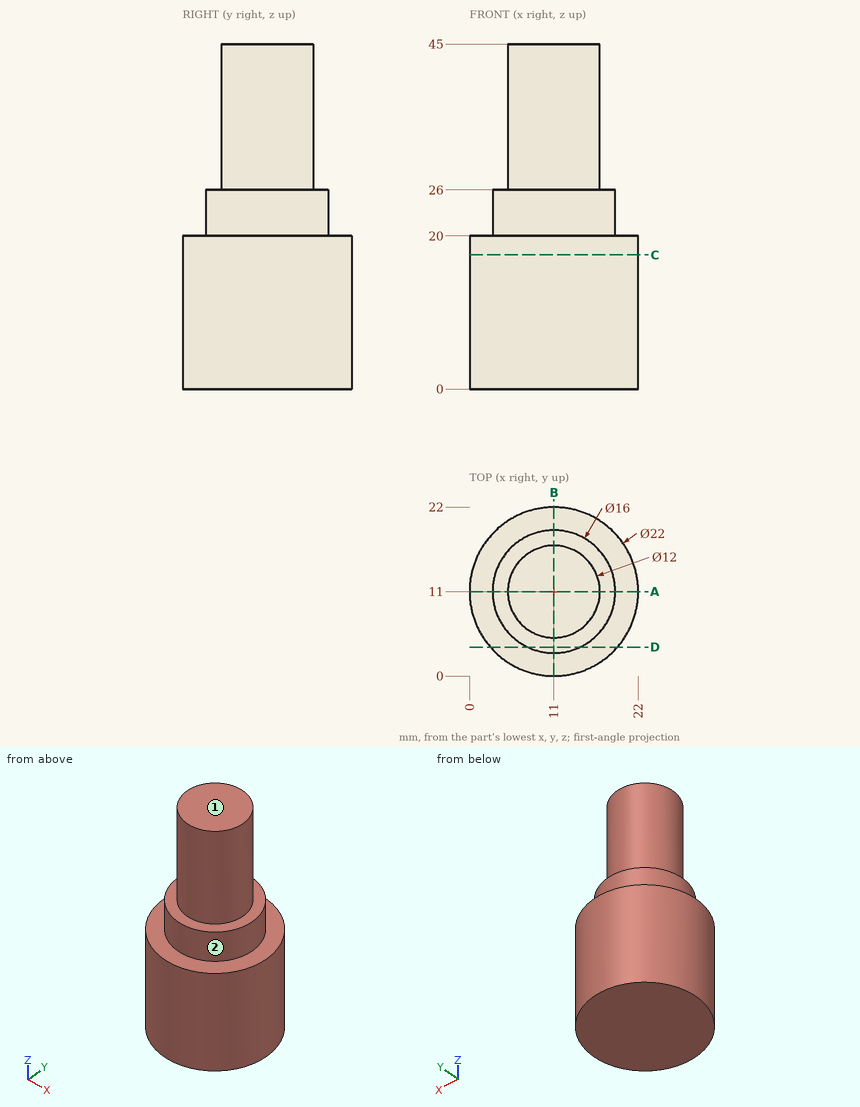
Job drawing, mm, ordinate dimensions from the low corner. One solid piece. A direction names the side the tool comes from. Round coordinates to 2 decimals unless told otherwise and drop trailing zeros. Write each loop counter-clockwise with the first axis right and the second up, starting at its lowest first coordinate (ties: lowest second). Pieces come first, ordered by that corner, then holes. Notation, with made-up numbers: (5.25, 47.5) -> (54.25, 47.5) arc R24 cw to (54.25, 76.5) -> close; hole circle Ø4 at (-31, 0.5). An arc over 180 degrees is marked (long way). Answer as a JSON object with one key per item and string values.
(1) Band-saw the part on D-D, the plane y = 3.75. List the corners of the cut face in (x, z), then the cut area to 3 significant figures.
Reported:
{"outline": "(2.73, 0) -> (19.27, 0) -> (19.27, 20) -> (14.38, 20) -> (14.38, 26) -> (7.62, 26) -> (7.62, 20) -> (2.73, 20) -> close", "area": "371 mm^2"}
(2) Band-saw the part on A-A, the plane y = 11. List the corners of the cut face in (x, z), then the cut area to 3 significant figures.
Reported:
{"outline": "(0, 0) -> (22, 0) -> (22, 20) -> (19, 20) -> (19, 26) -> (17, 26) -> (17, 45) -> (5, 45) -> (5, 26) -> (3, 26) -> (3, 20) -> (0, 20) -> close", "area": "764 mm^2"}
(3) Probe probe 1 along Z at (x, y) = (1.75, 16); probe 2 along Z at (x, y) = (11.5, 3.5); probe 3 along X at (y, z) = (10.25, 29.5). List the from-to ranges inside material, lowest first. Write a range as [from, to].
Reported:
{"probe 1": "z = [0, 20]", "probe 2": "z = [0, 26]", "probe 3": "x = [5.05, 16.95]"}
(4) Which spindle directions (+Z, -Z, +X, -X, +Y, -Y) get a long thin tool onto all of the face, cutting with end or side? Do the marked faces 1 and 2. Say none if no direction does.
Reported:
{"face 1": "+Z, +X, -X, +Y, -Y", "face 2": "+Z"}
(5) Band-saw the part on C-C, the plane z = 17.5. List the corners of the cut face in (x, y).
Reported:
{"outline": "circle Ø22 at (11, 11)"}
(6) Pin check, flat tips, straight feed: P1, Ø1, axis at y = 7, z = 5.5, coming from the +X side; P2, Ø4, axis at x = 14, z = 38, coming from the +Y side; P3, Ø1.5, axis at y = 14.5, z = 27.5, coming from the +X side. Stop position of each tip, or through.
Reported:
{"P1": "stops at x = 21.43", "P2": "stops at y = 16.92", "P3": "stops at x = 16.33"}
